Work out the finished part from the listing and answer in its coordinate system (mm). Face numbers are marked on the shaded views. A direction names the side the tool comes from. Give positions to 0.01 mm unless a question says otherwise; leave off trailing zeros. Loops run counter-clockwise (first coordinate to the right, second up) from the corner with the lowest first, then second, coordinate; pieces in that order, holes last.
from build123d import *

# Parameters (mm, degrees)
SKETCH1_R              = 23
BOSS_EXTRUDE1_DEPTH    = 18
SKETCH2_R              = 18
BOSS_EXTRUDE2_DEPTH    = 20
SKETCH3_R              = 8
CUT_EXTRUDE1_DEPTH     = 8
SKETCH4_R              = 10
CUT_EXTRUDE2_DEPTH     = 20
F_10_0MM_DOWEL_SLOT1_D = 10


with BuildPart() as part:
    # Sketch1 → Boss-Extrude1 (new body)
    with BuildSketch(Plane(origin=(0, 0, 0), x_dir=(1, 0, 0), z_dir=(0, 1, 0))):
        with Locations(Location((0, 0, 0), (0, 0, 270))):
            Circle(SKETCH1_R)
    extrude(amount=BOSS_EXTRUDE1_DEPTH)

    # Sketch2 → Boss-Extrude2 (add)
    with BuildSketch(Plane(origin=(0, 18, 0), x_dir=(1, 0, 0), z_dir=(0, 1, 0))):
        with Locations(Location((0, 0, 0), (0, 0, 270))):
            Circle(SKETCH2_R)
    extrude(amount=BOSS_EXTRUDE2_DEPTH)

    # Sketch3 → Cut-Extrude1 (cut)
    with BuildSketch(Plane(origin=(0, 0, 0), x_dir=(-1, 0, 0), z_dir=(0, -1, 0))):
        with Locations(Location((0, 0, 0), (0, 0, 90))):
            Circle(SKETCH3_R)
    extrude(amount=-CUT_EXTRUDE1_DEPTH, mode=Mode.SUBTRACT)

    # Sketch4 → Cut-Extrude2 (cut)
    with BuildSketch(Plane(origin=(0, 38, 0), x_dir=(1, 0, 0), z_dir=(0, 1, 0))):
        with Locations(Location((0, 0, 0), (0, 0, 270))):
            Circle(SKETCH4_R)
    extrude(amount=-CUT_EXTRUDE2_DEPTH, mode=Mode.SUBTRACT)

    # Ø10.0mm Dowel Slot1 (through all)
    with Locations(Plane(origin=(0, 18, 0), x_dir=(1, 0, 0), z_dir=(0, 1, 0))):
        with Locations((0, 0)):
            Hole(F_10_0MM_DOWEL_SLOT1_D / 2)


solid = part.part
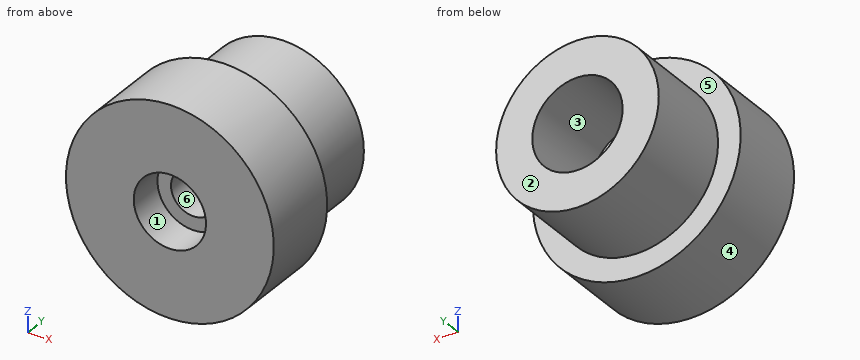
Item 1: Flat-ended cylindrical pins translate along their axes: pin 1 Ø12 at (x, y) = (10, 19) entering from +Z; pin 2 Ø1.5 at (x, y) = (-11.5, 16.5) entering from -Z; pin 3 Ø2 at (y, z) = (20.5, -13) entering from +X. Find the tip coordinate at first contact, or state that the pin passes through.
Item 2: Find section C-C, the plane y = 28.5. Write down the section's boundary in (x, z), plus the area to 3 significant figures.
Item 3: For the marked faces 1, 2 and 3, determine the directions among +Z, -Z, +X, -X, +Y, -Y from which every point of the face is accessible in a straight line to the end or side of a thin tool.
Item 4: Find section B-B, the plane z = 0. Write down the section's boundary in (x, y).
Item 5: Consider line 1 (X direction, y = 31, z = 0); line 2 (Z direction, x = 6.5, y = 27.5); line 3 (X direction, y = 23, z = 3.5). Determine where each line is inside the solid, lowest interval first.
Item 6: Find section A-A, the plane x = 0. Write down the section's boundary in (y, z), plus the area to 3 significant figures.
Item 7: Determine the mould class of the marked faces 4, 5 and 6 for opening direction X: released by +X, released by -X, zero draft, split by the parting line, or undercut.
Item 8: Find section D-D, the plane x = -16. Write down the section's boundary in (y, z).
Ans:
1. pin 1: stops at z = 22.63
1. pin 2: stops at z = -20.33
1. pin 3: stops at x = 13.42
2. outline: circle Ø36 at (0, 0); hole circle Ø20 at (0, 0)
2. area: 704 mm2
3. face 1: -Y
3. face 2: +Z, -Z, +X, -X, +Y
3. face 3: +Y
4. outline: (-23, 0) - (-8, 0) - (-8, 8) - (-5, 8) - (-5, 18) - (-10, 18) - (-10, 38) - (-18, 38) - (-18, 18) - (-23, 18) - close; (5, 8) - (8, 8) - (8, 0) - (23, 0) - (23, 18) - (18, 18) - (18, 38) - (10, 38) - (10, 18) - (5, 18) - close
5. line 1: x = -18 to -10, 10 to 18
5. line 2: z = -16.79 to -7.6, 7.6 to 16.79
5. line 3: x = -17.66 to -9.37, 9.37 to 17.66
6. outline: (0, -23) - (18, -23) - (18, -18) - (38, -18) - (38, -10) - (18, -10) - (18, -5) - (8, -5) - (8, -8) - (0, -8) - close; (0, 8) - (8, 8) - (8, 5) - (18, 5) - (18, 10) - (38, 10) - (38, 18) - (18, 18) - (18, 23) - (0, 23) - close
6. area: 920 mm2
7. face 4: split by the parting line
7. face 5: zero draft
7. face 6: undercut
8. outline: (0, -16.52) - (18, -16.52) - (18, -8.25) - (38, -8.25) - (38, 8.25) - (18, 8.25) - (18, 16.52) - (0, 16.52) - close
